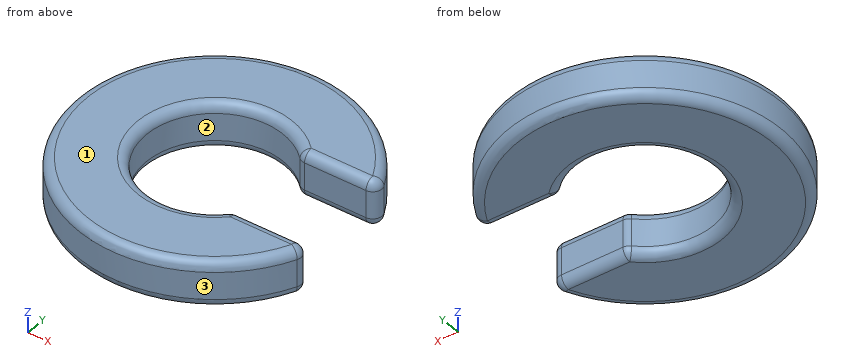
```python
from build123d import *

# Parameters (mm, degrees)
BOX_W             = 3
BOX_H             = 2
BOX_DEPTH         = 10
CYLINDER_R        = 1.5
CYLINDER_DEPTH    = 1
CYLINDER001_R     = 3
CYLINDER001_DEPTH = 1
FILLET_R          = 0.2


with BuildPart() as cube:
    # Box → Box (new body)
    with BuildSketch(Plane(origin=(0, -1, 0), x_dir=(1, 0, 0), z_dir=(0, 0, 1))):
        with Locations((1.5, 1)):
            Rectangle(BOX_W, BOX_H)
    extrude(amount=BOX_DEPTH)


with BuildPart() as cylinder:
    # Cylinder → Cylinder (new body)
    with BuildSketch(Plane.XY):
        Circle(CYLINDER_R)
    extrude(amount=CYLINDER_DEPTH)


with BuildPart() as obj1:
    # Cylinder001 → Cylinder001 (new body)
    with BuildSketch(Plane.XY):
        Circle(CYLINDER001_R)
    extrude(amount=CYLINDER001_DEPTH)

    # Cut: cut Cylinder
    add(cylinder.part, mode=Mode.SUBTRACT)

    # Cut001: cut Cube
    add(cube.part, mode=Mode.SUBTRACT)

    # Fillet
    fillet_edges = [obj1.edges().sort_by_distance(p)[0] for p in [
        (-3, 0, 0),
        (2.828427, -1, 0.5),
        (-3, 0, 1),
        (2.828427, 1, 0.5),
        (1.973231, 1, 0),
        (-1.5, 0, 0),
        (1.973231, -1, 0),
        (1.973231, -1, 1),
        (1.118034, -1, 0.5),
        (1.973231, 1, 1),
        (-1.5, 0, 1),
        (1.118034, 1, 0.5),
    ]]
    fillet(fillet_edges, radius=FILLET_R)


solid = obj1.part
```
Source: CAD feature listing. Evaluate the final solid. Frame: model axes, mm. Face numbers are marked on the shaded views. Give positions to 0.01 mm unless a question says otherwise; leave off trailing zeros. Write each loop counter-clockwise with the first axis right and the second up, starting at its lowest first coordinate (ties: lowest second). Pieces come first, ordered by that corner, then holes. Notation, with made-up numbers: (88.25, 71) - (110.25, 71) arc R29 cw to (110.25, 104) - close; hole circle Ø7 at (83.5, 72.25). An arc over 180 degrees is marked (long way). One line per item, written item: value. Start each with the question number.
Q1. Material intervals for probe 1 along Y at (x, z) = (0, 0.4); probe 2 along Z at (x, y) = (0.75, 1.5); probe 3 along Y at (x, z) = (0.6, 0.55), sorted ascending. Write a range as from..to.
Q2. Section query B-B, the plane y = 0. Return the cut outline in (x, z), then the cut area to 3 significant figures.
Q3. Section query A-A, the plane x = 0. Return the cut outline in (y, z).
Q4. Draft query along X for the marked faces 1, 2 and 3. Return one class per face: +X half, -X half, draft (parallel to the pull), parting line (faces both ways), or undercut.
Q5. Section query C-C, the plane z = 0.6. Return the cut outline in (x, y).
Q6. First-contact query: pin 1 Ø1.5 at (x, y) = (0.5, -1.5) entering from -Z. Flat tip, straight axial feed; report the tip coordinate or a pass-through.
Answer:
1. probe 1: y = -3..-1.5, 1.5..3
1. probe 2: z = 0..1
1. probe 3: y = -2.94..-1.37, 1.37..2.94
2. outline: (-3, 0.2) arc R0.2 ccw to (-2.8, 0) - (-1.7, 0) arc R0.2 ccw to (-1.5, 0.2) - (-1.5, 0.8) arc R0.2 ccw to (-1.7, 1) - (-2.8, 1) arc R0.2 ccw to (-3, 0.8) - close
2. area: 1.47 mm2
3. outline: (-3, 0.2) arc R0.2 ccw to (-2.8, 0) - (-1.7, 0) arc R0.2 ccw to (-1.5, 0.2) - (-1.5, 0.8) arc R0.2 ccw to (-1.7, 1) - (-2.8, 1) arc R0.2 ccw to (-3, 0.8) - close; (1.5, 0.2) arc R0.2 ccw to (1.7, 0) - (2.8, 0) arc R0.2 ccw to (3, 0.2) - (3, 0.8) arc R0.2 ccw to (2.8, 1) - (1.7, 1) arc R0.2 ccw to (1.5, 0.8) - close
4. face 1: draft
4. face 2: undercut
4. face 3: parting line
5. outline: (1.06, -1.06) arc R1.5 cw (long way) to (1.06, 1.06) arc R0.2 ccw to (1.2, 1) - (2.53, 1) arc R0.2 ccw to (2.71, 1.29) arc R3 ccw (long way) to (2.71, -1.29) arc R0.2 ccw to (2.53, -1) - (1.2, -1) arc R0.2 ccw to start
6. pin 1: stops at z = 0
